Here's how the part is built. I have some questions about the finished solid (model axes, mm). A direction names the side the tool comes from. Round coordinates to 2 decimals unless told otherwise and drop trailing zeros. Loops run counter-clockwise (first coordinate to the right, second up) from the corner with the lowest first, then second, coordinate; pieces in that order, holes last. Notation, with made-up numbers: M 28,18.5 L 67,18.5 A18 ccw 67,41.5 Z; hole C 17,31 d6. An arc over 180 degrees is marked long. Write each question's results on one line, items separated by ' | '. Start each with the question number.
```python
from build123d import *

# Parameters (mm, degrees)
SKETCH1_W           = 457.2
SKETCH1_H           = 254
BOSS_EXTRUDE1_DEPTH = 101.6
SHELL1_T            = -6.35
FILLET1_R           = 5.08
CUT_EXTRUDE1_REACH  = 358.506
SKETCH3_W           = 39.624
SKETCH3_H           = 39.624
CUT_EXTRUDE3_REACH  = 358.506
SKETCH6_R           = 3.175
CUT_EXTRUDE4_REACH  = 358.506
SKETCH7_W           = 26.67
SKETCH7_H           = 18.796


with BuildPart() as part:
    # Sketch1 → Boss-Extrude1 (new body)
    with BuildSketch(Plane(origin=(0, 0, 0), x_dir=(1, 0, 0), z_dir=(0, 1, 0))):
        Rectangle(SKETCH1_W, SKETCH1_H)
    extrude(amount=BOSS_EXTRUDE1_DEPTH)

    # Shell1
    shell1_openings = [part.faces().sort_by_distance(p)[0] for p in [
        (0, 101.6, 0),
    ]]
    offset(amount=SHELL1_T, openings=shell1_openings, kind=Kind.INTERSECTION)

    # Fillet1
    fillet1_edges = [part.edges().sort_by_distance(p)[0] for p in [
        (228.6, 101.6, 0),
        (0, 101.6, -127),
        (-228.6, 101.6, 0),
        (0, 101.6, 127),
        (-228.6, 50.8, -127),
        (228.6, 50.8, -127),
        (228.6, 50.8, 127),
        (-228.6, 50.8, 127),
    ]]
    fillet(fillet1_edges, radius=FILLET1_R)

    # Sketch3 → Cut-Extrude1 (cut, up to next)
    with BuildSketch(Plane.XY.offset(127), mode=Mode.PRIVATE) as cut_extrude1_sk1:
        with Locations((0, 48.26)):
            Rectangle(SKETCH3_W, SKETCH3_H)
    cut_extrude1_tool1 = extrude(cut_extrude1_sk1.sketch, amount=-CUT_EXTRUDE1_REACH, mode=Mode.PRIVATE) & part.part
    add(cut_extrude1_tool1.solids().sort_by_distance((0, 48.26, 127))[0], mode=Mode.SUBTRACT)

    # Sketch6 → Cut-Extrude3 (cut, up to next)
    with BuildSketch(Plane(origin=(0, 0, -127), x_dir=(-1, 0, 0), z_dir=(0, 0, -1)), mode=Mode.PRIVATE) as cut_extrude3_sk1:
        with Locations((147.32, 65.278)):
            Circle(SKETCH6_R)
    cut_extrude3_tool1 = extrude(cut_extrude3_sk1.sketch, amount=-CUT_EXTRUDE3_REACH, mode=Mode.PRIVATE) & part.part
    # Sketch6 → Cut-Extrude3 (cut, up to next)
    with BuildSketch(Plane(origin=(0, 0, -127), x_dir=(-1, 0, 0), z_dir=(0, 0, -1)), mode=Mode.PRIVATE) as cut_extrude3_sk2:
        with Locations((110.744, 65.278)):
            Circle(SKETCH6_R)
    cut_extrude3_tool2 = extrude(cut_extrude3_sk2.sketch, amount=-CUT_EXTRUDE3_REACH, mode=Mode.PRIVATE) & part.part
    # Sketch6 → Cut-Extrude3 (cut, up to next)
    with BuildSketch(Plane(origin=(0, 0, -127), x_dir=(-1, 0, 0), z_dir=(0, 0, -1)), mode=Mode.PRIVATE) as cut_extrude3_sk3:
        with Locations(Location((-147.32, 65.278, 0), (0, 0, 180))):
            Circle(SKETCH6_R)
    cut_extrude3_tool3 = extrude(cut_extrude3_sk3.sketch, amount=-CUT_EXTRUDE3_REACH, mode=Mode.PRIVATE) & part.part
    # Sketch6 → Cut-Extrude3 (cut, up to next)
    with BuildSketch(Plane(origin=(0, 0, -127), x_dir=(-1, 0, 0), z_dir=(0, 0, -1)), mode=Mode.PRIVATE) as cut_extrude3_sk4:
        with Locations(Location((-110.744, 65.278, 0), (0, 0, 180))):
            Circle(SKETCH6_R)
    cut_extrude3_tool4 = extrude(cut_extrude3_sk4.sketch, amount=-CUT_EXTRUDE3_REACH, mode=Mode.PRIVATE) & part.part
    add(cut_extrude3_tool1.solids().sort_by_distance((-147.32, 65.278, -127))[0], mode=Mode.SUBTRACT)
    add(cut_extrude3_tool2.solids().sort_by_distance((-110.744, 65.278, -127))[0], mode=Mode.SUBTRACT)
    add(cut_extrude3_tool3.solids().sort_by_distance((147.32, 65.278, -127))[0], mode=Mode.SUBTRACT)
    add(cut_extrude3_tool4.solids().sort_by_distance((110.744, 65.278, -127))[0], mode=Mode.SUBTRACT)

    # Sketch7 → Cut-Extrude4 (cut, up to next)
    with BuildSketch(Plane(origin=(0, 0, -127), x_dir=(-1, 0, 0), z_dir=(0, 0, -1)), mode=Mode.PRIVATE) as cut_extrude4_sk1:
        with Locations((172.085, 34.798)):
            Rectangle(SKETCH7_W, SKETCH7_H)
    cut_extrude4_tool1 = extrude(cut_extrude4_sk1.sketch, amount=-CUT_EXTRUDE4_REACH, mode=Mode.PRIVATE) & part.part
    add(cut_extrude4_tool1.solids().sort_by_distance((-172.085, 34.798, -127))[0], mode=Mode.SUBTRACT)


solid = part.part
```
1. Which directions (+Z, -Z, +X, -X, +Y, -Y) give clear straight access to the entire face, cutting with the end or side of a thin tool? Please do faces 1 (the face through (-3, 53, -120.65)), 2 (the face through (-3, 69, 127)).
2. For pin 1 (6 mm diameter, centred on x = -73, z = 0, fed in from +Y); pin 2 (5.5 mm diameter, centred on x = -147.32, y = 65.278, fed in from -Z); pin 3 (3 mm diameter, centred on x = 9, z = 124.5, fed in from +Y), each with a flat end and sliding along its axis, tell me the tip position at first contact or that it passes through.
3. If we mould it in two halves opening along Z, with no side actions, what happens to faces 3 (the face through (-3, 6.35, -2)), 4 (the face through (-3, 0, -2)), 5 (the face through (-3, 48, -127))? For each: released by +Z, released by -Z, zero draft, split by the parting line, or undercut.
4. I want a section at B-B on x = 94. List the corners of the cut face in (y, z) for me, plus the area to 3 significant figures.
5. I want a section at C-C on y = 14.5. List the corners of the cut face in (x, z) for me, plus the area to 3 significant figures.
6. I want a section at A-A on y = 37. List the corners of the cut face in (x, z) for me, plus the area to 3 significant figures.
7. I need wall thicknesses on line 1 along Z through (x, y) = (-150, 87); line 2 along Y through (x, z) = (147, -122); line 3 along X through (y, z) = (34, 70). Which ranges of each line are inside material? Lowest first, please.
8. I want a section at D-D on z = 109. List the corners of the cut face in (x, y) for me.
Outcome:
1) face 1: +Y | face 2: +Z, +X, -X, +Y, -Y
2) pin 1: y = 6.35 | pin 2: z = 120.65 | pin 3: y = 101.48
3) face 3: undercut | face 4: zero draft | face 5: released by -Z
4) outline: M 0,-127 L 96.52,-127 A5.08 ccw 101.6,-121.92 L 101.6,-120.65 L 6.35,-120.65 L 6.35,120.65 L 101.6,120.65 L 101.6,121.92 A5.08 ccw 96.52,127 L 0,127 Z | area: 2,810 mm2
5) outline: M -228.6,-121.92 A5.08 ccw -223.52,-127 L 223.52,-127 A5.08 ccw 228.6,-121.92 L 228.6,121.92 A5.08 ccw 223.52,127 L -223.52,127 A5.08 ccw -228.6,121.92 Z; hole M -222.25,-120.65 L 222.25,-120.65 L 222.25,120.65 L -222.25,120.65 Z | area: 8,850 mm2
6) outline: M -228.6,-121.92 A5.08 ccw -223.52,-127 L -185.42,-127 L -185.42,-120.65 L -222.25,-120.65 L -222.25,120.65 L -19.81,120.65 L -19.81,127 L -223.52,127 A5.08 ccw -228.6,121.92 Z; M -158.75,-127 L 223.52,-127 A5.08 ccw 228.6,-121.92 L 228.6,121.92 A5.08 ccw 223.52,127 L 19.81,127 L 19.81,120.65 L 222.25,120.65 L 222.25,-120.65 L -158.75,-120.65 Z | area: 8,430 mm2
7) line 1: -127 to -120.65, 120.65 to 127 | line 2: 0 to 62.12, 68.44 to 101.6 | line 3: -228.6 to -222.25, 222.25 to 228.6
8) outline: M -228.6,0 L 228.6,0 L 228.6,96.52 A5.08 ccw 223.52,101.6 L 222.25,101.6 L 222.25,6.35 L -222.25,6.35 L -222.25,101.6 L -223.52,101.6 A5.08 ccw -228.6,96.52 Z
